Check sheet for the modelled part. Datum: model origin and axes. Units: mm. Give positions to 0.01 mm unless a question says otherwise; leave off trailing zeros. Loops run counter-clockwise (first coordinate to the right, second up) from the corner with the lowest first, then second, coordinate; pieces in that order, holes last. Notation, with made-up numbers: (29.5, 40) - (62.5, 40) arc R25 cw to (62.5, 78) - close; hole circle Ø7 at (40, -26.75). An arc over 180 degrees is marked (long way). Use CSV: the item, a comma, the result in double quotes.
from build123d import *

# Parameters (mm, degrees)
F0_W     = 101.6
F0_H     = 101.6
F1_DEPTH = 50.8
F3_D     = 6.35


with BuildPart() as f1:
    # F0 (on Front) → F1 (new body, symmetric)
    with BuildSketch(Plane.XZ):
        Rectangle(F0_W, F0_H)
    extrude(amount=F1_DEPTH, both=True)

    # F3 (through all)
    with Locations(Plane.XY.offset(50.8)):
        with Locations((0, 0)):
            Hole(F3_D / 2)


solid = f1.part
1. Sectioned sample at A-A, the plane x = 0. Record the boundary of the cut face in (y, z) (3 decimals), and give its area (3 significant figures).
Completed:
outline,"(-50.8, -50.8) - (-3.175, -50.8) - (-3.175, 50.8) - (-50.8, 50.8) - close; (3.175, -50.8) - (50.8, -50.8) - (50.8, 50.8) - (3.175, 50.8) - close"
area,"9,680 mm²"
2. Release check for a two-part mould opening along X. For faces 1 (the face through (0.69, -3.1, -0.71)), 2 (the face through (50.8, -1, -1)), 3 (the face through (11, -1, 50.8)) record: released by +X, released by -X, zero draft, split by the parting line, or undercut.
Completed:
face 1,"undercut"
face 2,"released by +X"
face 3,"zero draft"
3. Scan lines: line 1 along Y through (x, z) = (0, -17.5) (3 decimals); line 2 along X through (y, z) = (1.5, -40); line 3 along X through (y, z) = (2, -38.5). Record each from-to range of solid material in increasing order.
Completed:
line 1,"y = -50.8 to -3.175, 3.175 to 50.8"
line 2,"x = -50.8 to -2.8, 2.8 to 50.8"
line 3,"x = -50.8 to -2.47, 2.47 to 50.8"
